from build123d import *

# Parameters (mm, degrees)
F1_DEPTH = 12.7
F2_R     = 12.7
F3_DEPTH = 12.7
F4_W     = 50.8
F4_H     = 12.7
F5_DEPTH = 38.1
F6_W     = 12.7
F6_H     = 12.7
F7_DEPTH = 39.998543


with BuildPart() as f1:
    # F0 (on Front) → F1 (new body)
    with BuildSketch(Plane.XZ):
        with BuildLine():
            ThreePointArc((26.159194, 36.202457), (0.759194, 61.602457), (-24.640806, 36.202457))
            Line((-24.640806, 36.202457), (26.159194, 36.202457))
        make_face()
        with BuildLine():
            ThreePointArc((26.159194, 36.202457), (0.759194, 10.802457), (-24.640806, 36.202457))
            Line((-24.640806, 36.202457), (-24.640806, -39.997543))
            Line((-24.640806, -39.997543), (26.159194, -39.997543))
            Line((26.159194, -39.997543), (26.159194, 36.202457))
        make_face()
        with BuildLine():
            Line((26.159194, 36.202457), (-24.640806, 36.202457))
            ThreePointArc((-24.640806, 36.202457), (0.759194, 10.802457), (26.159194, 36.202457))
        make_face()
    extrude(amount=F1_DEPTH)

    # F2 (on Front) → F3 (cut)
    with BuildSketch(Plane.XZ):
        with Locations((0, 46.423854)):
            Circle(F2_R)
    extrude(amount=F3_DEPTH, mode=Mode.SUBTRACT)

    # F4 (on Front) → F5 (join)
    with BuildSketch(Plane.XZ):
        with Locations((0.759194, -33.647543)):
            Rectangle(F4_W, F4_H)
    extrude(amount=F5_DEPTH)

    # F6 (on Top) → F7 (cut, through all)
    with BuildSketch(Plane.XY):
        with Locations((19.809194, -31.75)):
            Rectangle(F6_W, F6_H)
    extrude(amount=-F7_DEPTH, mode=Mode.SUBTRACT)


solid = f1.part
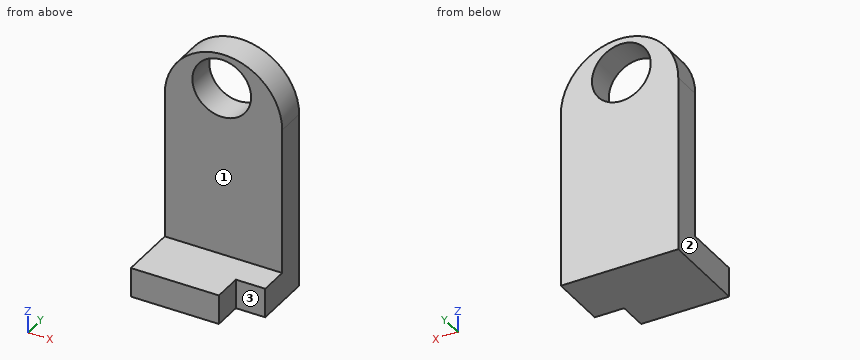
Verification items for the finished model (mm, model axes). Face numbers are marked on the shaded views. A direction names the side the tool comes from. Coordinates: 2 decimals unless noted, no trailing zeros. Loops run counter-clockwise (first coordinate to the right, second up) from the corner with the lowest first, then second, coordinate; pieces in that order, holes last. Notation, with made-up numbers: M -10,47 L 18,47 A11 ccw 18,67 Z; hole C 55,8.25 d7. An arc over 180 degrees is marked long. One line per item, written item: value.
1. Section check D-D on x = 18. Record the cut outline in (y, z).
Answers follow:
outline: M -25.4,-40 L 0,-40 L 0,54.85 L -12.7,54.85 L -12.7,-27.3 L -25.4,-27.3 Z
2. Set-up check for the marked faces 1, 2 and 3: record each of +Z, -Z, +X, -X, +Y, -Y from which the full face is reachable in a straight line by a thin tool's end or side.
Answers follow:
face 1: +Z, +X, -X, -Y
face 2: +Z, -Z, -X, +Y, -Y
face 3: +Z, -Z, +X, -Y
3. Section check C-C on y = -9.5. Record the cut outline in (x, z), plus the area to 3 significant figures.
Answers follow:
outline: M -24.64,-40 L 26.16,-40 L 26.16,36.2 A25.4 ccw -24.64,36.2 Z; hole C 0,46.42 d25.4
area: 4,380 mm^2
4. Material ranges on line 1 along Z through (x, y) = (0, -5.75); line 2 along X through (y, z) = (-26.5, -35); line 3 along Y through (x, z) = (18.5, 32.5), recorded low to high. Write a range as from..to.
Answers follow:
line 1: -40..33.72, 59.12..61.59
line 2: -24.64..13.46
line 3: -12.7..0
5. Section check B-B on z = 53.5. Record the cut outline in (x, y).
Answers follow:
outline: M -17.84,-12.7 L -10.55,-12.7 L -10.55,0 L -17.84,0 Z; M 10.55,-12.7 L 19.36,-12.7 L 19.36,0 L 10.55,0 Z
6. Section check A-A on x = 7. Record the cut outline in (y, z), plus the area to 3 significant figures.
Answers follow:
outline: M -38.1,-40 L 0,-40 L 0,35.83 L -12.7,35.83 L -12.7,-27.3 L -38.1,-27.3 Z; M -12.7,57.02 L 0,57.02 L 0,60.82 L -12.7,60.82 Z
area: 1,330 mm^2
7. Gauge pin test, flat ends, axial feed: P1, Ø3, axis at x = 19, y = -12.5, coming from the +Z side; P2, Ø1, axis at x = 10.5, z = 25, coming from the -Y side; P3, Ø4, axis at x = 22, z = -31.5, coming from the -Y side. Record the tip position at first contact, or that the pin passes through.
Answers follow:
P1: z = 55.3
P2: y = -12.7
P3: y = -25.4
